Autodesk Inventor part; units mm, degrees
ref_plane "YZ Plane" through (0, 0, 0) normal (1, 0, 0) x (0, 1, 0)
ref_plane "XZ Plane" through (0, 0, 0) normal (0, 1, 0) x (-1, 0, 0)
ref_plane "XY Plane" through (0, 0, 0) normal (0, 0, 1) x (1, 0, 0)
sketch "Sketch19" plane through (0, 0, 0) normal (1, 0, 0) x (0, 1, 0)
  line L0 (0, 0) -> (0, -22)
  line L1 (0, -22) -> (3.4577, -59.4814)
  line L2 (3.5, -60.4) -> (3.5, -85)
  line L3 (3.5, -85) -> (10.5, -85)
  line L4 (10.5, -85) -> (10.5, -60.4)
  line L5 (10.4577, -59.4814) -> (7, -22)
  line L6 (7, -22) -> (7, 0)
  line L7 (7, 0) -> (0, 0)
  arc A0 (3.5, -60.4) -> (3.4577, -59.4814) centre (-6.5, -60.4) ccw
  arc A1 (10.5, -60.4) -> (10.4577, -59.4814) centre (0.5, -60.4) ccw
  point P0 (10.4894, -59.9402)
  dimension "d79" = 10
  dimension "d80" = 10
  dimension "d82" = 7
  dimension "d83" = 3.5
  dimension "d84" = 24.6
  dimension "d85" = 22
  dimension "d86" = 37.9402
extrude "Extrusion7" add sketch "Sketch19" along normal blind 12
sketch "Sketch20" plane through (0, 7, 0) normal (0, 1, 0) x (1, 0, 0)
  circle A0 centre (6, 6) radius 6
  line L0 (0, 0) -> (12, 0)
  line L1 (0, 0) -> (12, 0)
  line L2 (0, 0) -> (0, 6)
  line L3 (0, 0) -> (0, 22)
  line L4 (12, 0) -> (12, 6)
  point P0 (6, 0)
  point P1 (6, 0)
  dimension "d89" = 12
extrude "Extrusion8" cut sketch "Sketch20" against normal blind 12 contours L4 L0 A0 | A0 L0 L2
sketch "Sketch21" plane through (0, 10.5, -60.4) normal (0, 1, 0) x (1, 0, 0)
  circle A0 centre (6, 20.6) radius 4
  line L0 (0, 24.6) -> (12, 24.6)
  arc A1 (0, -54.4) -> (12, -54.4) centre (6, -54.4) ccw
  line L1 (12, -38.4) -> (12, -54.4)
  line L2 (0, -38.4) -> (12, -38.4)
  line L3 (0, -38.4) -> (0, -54.4)
  line L4 (0, -38.4) -> (2.0023, 20.7354)
  line L5 (12, -38.4) -> (12, -0.9186)
  line L6 (12, -38.4) -> (9.9977, 20.7354)
  line L7 (0, 24.6) -> (0, 0)
  line L8 (0, -38.4) -> (0, 24.6)
  line L9 (0, 24.6) -> (6, 24.6)
  line L10 (6, 24.6) -> (12, 24.6)
  line L11 (12, 0) -> (12, 24.6)
  line L12 (12, 24.6) -> (12, -38.4)
  point P0 (0, -60.4)
  point P1 (12, 0)
  dimension "d93" = 8
extrude "Extrusion9" cut sketch "Sketch21" against normal up to surface (10.5 mm away) contours A0 L0 L11 L12 L5 L6 | L4 L8 L7 L0 A0
sketch "Sketch22" plane through (6, 7, -6) normal (0, 1, 0) x (1, 0, 0)
  arc A0 (-6, 0) -> (6, 0) centre (0, 0) ccw
  point P0 (-6, -6)
hole "Hole1" at (6, 7, -6) direction (0, -1, 0) diameter 10 end through all
sketch "Sketch23" plane through (6, 10.5, -81) normal (0, 1, 0) x (1, 0, 0)
  arc A0 (3.9977, 0.1354) -> (-3.9977, 0.1354) centre (0, 0) ccw
  point P0 (-6, -81)
hole "Hole2" at (6, 10.5, -81) direction (0, -1, 0) diameter 5 end through all
fillet "Fillet1" radius 10 1 edges at (6, 7, -22)
properties part number "47"
The model under review builds one solid part; all positions refer to its coordinate system, in mm. A direction names the side the tool comes from. Give positions to 0.01 mm unless a question says otherwise; leave off trailing zeros. Order: outer loops, then holes, each group sorted by start corner. A loop starts at its lowest first (then second) coordinate and runs counter-clockwise, first axis right, second up. Notation, with made-up numbers: M -21.75,-1 L 9.25,-1 A25 ccw 9.25,22 Z; hole C -33.5,68.5 d9. An arc over 180 degrees is marked long. Answer in a Markdown table with one row per item. Add a question column.
1. Add section A-A on y = 5. State the section outline as (x, z) points.
2. To check wall thickness, follow line 1 along Z through (x, y) = (6, 6.75); line 2 along X through (y, z) = (5.25, -6); line 3 along Y through (x, z) = (3.75, -65). State the ranges of each line that lie inside material, in increasing order.
3. Mouldability with a two-part tool opening along Z and no side actions: class faces 3 (the flat face through (5.916, 1.705, -40.478)), 4 (the cylindrical face through (5.9, 7, -83.5)), 5 (the flat face through (6, 7, -13)) as released by +Z, released by -Z, zero draft, split by the parting line, or undercut.
4. For pin 1 Ø3 at (x, z) = (4, -68) entering from -Y; pin 2 Ø6 at (x, z) = (6, -6) entering from +Y; pin 3 Ø3 at (x, z) = (4.5, -38) entering from +Y; pin 4 Ø1 at (x, y) = (1.5, 2) entering from +Z, all flat-tipped, find the tip position at first contact; note any pin that passes through.
5. Machinability: for faces 1 (the flat face through (6, 0, -13)), 2 (the flat face through (6, 3.5, -70)), which of the approach directions +Z, -Z, +X, -X, +Y, -Y give a long, thin tool a straight path to every point of the face, cutting with its end or side? Answer none if there is none.
6. Add section B-B on x = 6. State the section outline as (y, z) points, plus the area to 3 significant figures.
7. Add section D-D on z = -28. State the section outline as (x, y) points.
8. Add section C-C on y = 8.25. State the section outline as (x, z) points, plus the area to 3 significant figures.
The answers:
| question | item | result |
|---|---|---|
| 1 | outline | M 0,-22 L 2,-81.14 A4 ccw 10,-81.14 L 12,-22 L 12,-6 A6 ccw 0,-6 Z; hole C 6,-6 d10; hole C 6,-81 d5 |
| 2 | line 1 | -85 to -83.5, -78.5 to -11, -1 to 0 |
| 2 | line 2 | 0 to 1, 11 to 12 |
| 2 | line 3 | 3.5 to 10.5 |
| 3 | face 3 | released by -Z |
| 3 | face 4 | undercut |
| 3 | face 5 | zero draft |
| 4 | pin 1 | y = 3.5 |
| 4 | pin 2 | through |
| 4 | pin 3 | y = 8.61 |
| 4 | pin 4 | z = -1.53 |
| 5 | face 1 | +Z, -Z, +X, -X, -Y |
| 5 | face 2 | -Z, +X, -X, -Y |
| 6 | outline | M 0,-22 L 3.46,-59.48 A9.99 cw 3.5,-60.4 L 3.5,-78.5 L 10.5,-78.5 L 10.5,-60.4 A9.99 ccw 10.46,-59.48 L 7.04,-22.46 A10 cw 7,-21.54 L 7,-11 L 0,-11 Z; M 0,-1 L 7,-1 L 7,0 L 0,0 Z; M 3.5,-85 L 10.5,-85 L 10.5,-83.5 L 3.5,-83.5 Z |
| 6 | area | 490 mm2 |
| 7 | outline | M 0.2,0.55 L 11.8,0.55 L 11.8,7.55 L 0.2,7.55 Z |
| 8 | outline | M 0.46,-35.55 L 2,-81.14 A4 ccw 10,-81.14 L 11.54,-35.55 Z; hole C 6,-81 d5 |
| 8 | area | 439 mm2 |
